Job drawing, mm, ordinate dimensions from the low corner. One solid piece. Give positions to 0.01 mm unless a question says otherwise; leave off trailing zeros. Order: outer loops, then holes, each group sorted by start corner. A loop starts at its lowest first (then second) coordinate and runs counter-clockwise, first axis right, second up. Notation, with made-up numbers: (54.5, -24) - (102.5, -24) arc R8 cw to (102.5, -12) - close; hole circle Ø6 at (72.5, -16). An arc over 180 degrees is marked (long way). Write each question's results on one line, items separated by ' | '. Start each with the question number.
1) Cut at A-A on z = 46.5. List the corners of the cut face in (x, y), plus the area to 3 significant figures.
2) Drill centre lines: line 1 along Z through (x, y) = (66, 2.2); line 2 along Z through (x, y) = (49.5, 2.45); line 3 along Z through (x, y) = (112, 2.9). Where is each one in solid material? Low to high. Write a range as from..to.
3) Cut at B-B on x = 74.5. List the corners of the cut face in (y, z), plus the area to 3 significant figures.
4) Drop flat-ended pins along their axis: pin 1 Ø0.9 at (x, y) = (61.5, 1.5) entering from -Z; pin 2 Ø1.4 at (x, y) = (65.5, 1) entering from +Z; pin 3 Ø0.9 at (y, z) = (2, 65.5) entering from +X. Give the stop position or say it passes through.
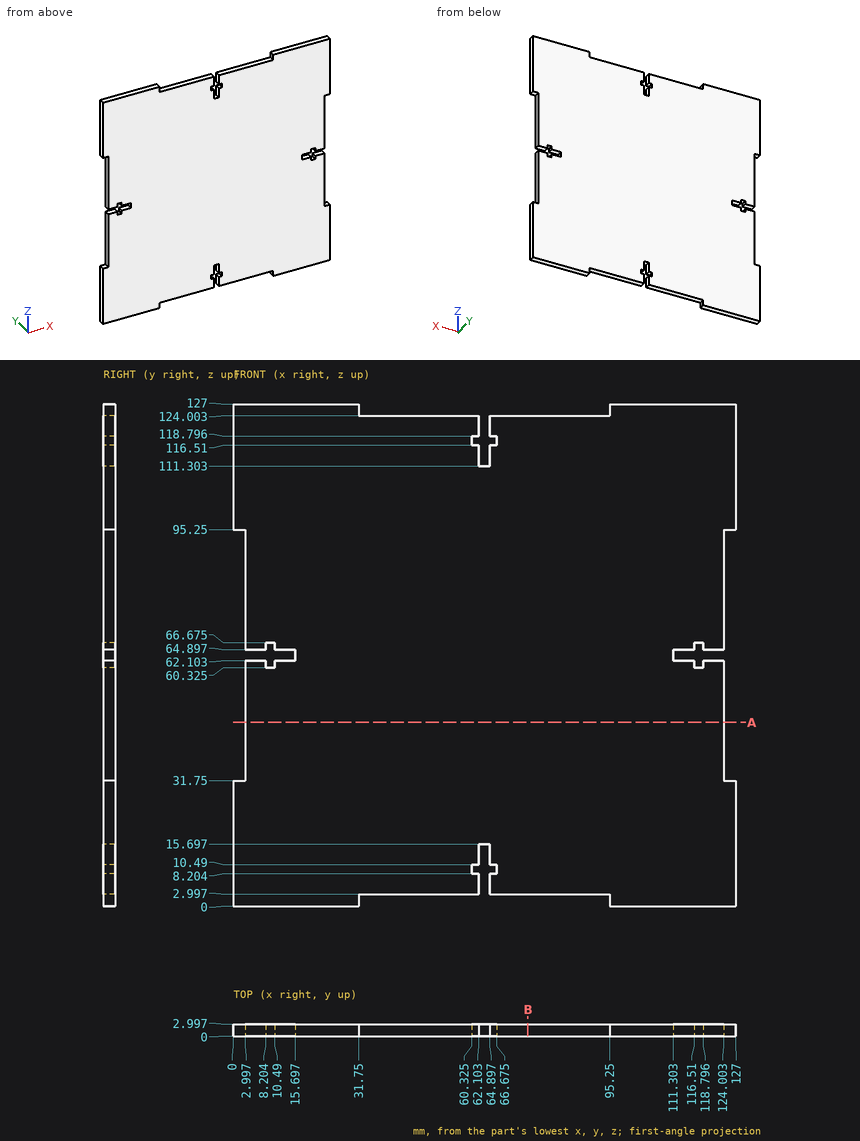
Results:
1) outline: (3, 0) - (124, 0) - (124, 3) - (3, 3) - close | area: 363 mm^2
2) line 1: 3..8.2, 10.49..116.51, 118.8..124 | line 2: 3..124 | line 3: 0..62.1, 64.9..127
3) outline: (0, 3) - (3, 3) - (3, 124) - (0, 124) - close | area: 363 mm^2
4) pin 1: z = 3 | pin 2: z = 124 | pin 3: x = 124
